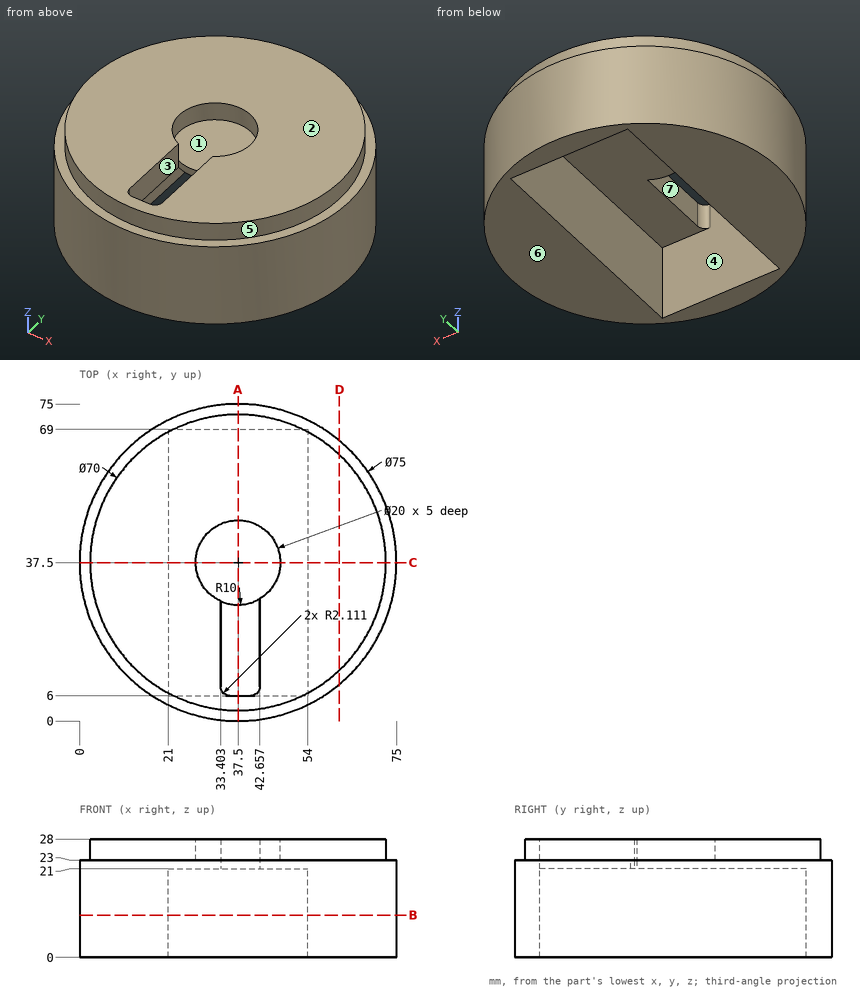
The drawing under review shows one solid part. Ordinate dimensions are in mm from its lowest x, y, z. A direction names the side the tool comes from. Coordinates: 2 decimals unless noted, no trailing zeros. Loops run counter-clockwise (first coordinate to the right, second up) from the corner with the lowest first, then second, coordinate; pieces in that order, holes last. Notation, with made-up numbers: M -40,20 L -14,20 A19 ccw -14,43 Z; hole C 87.25,69.25 d9. An arc over 180 degrees is marked long. Use one line per item in the form item = value.
(1) Consider section A-A (x = 37.5). Write out the cut boundary in (y, z).
Return value:
outline = M 0,0 L 6,0 L 6,28 L 2.5,28 L 2.5,23 L 0,23 Z; M 27.5,21 L 69,21 L 69,0 L 75,0 L 75,23 L 72.5,23 L 72.5,28 L 47.5,28 L 47.5,23 L 27.5,23 Z
(2) Consider section B-B (z = 10). Write out the cut boundary in (x, y), and give its area (3 significant figures).
Return value:
outline = C 37.5,37.5 d75; hole M 21,6 L 54,6 L 54,69 L 21,69 Z
area = 2,340 mm2
(3) Clearance check with flat-ended pins moving along their axes: P1, Ø12, axis at x = 37.5, y = 37.5, coming from the -Z side; P2, Ø2, axis at y = 19, z = 23.5, coming from the +X side (1 decimal); P3, Ø4, axis at y = 52.5, z = 8, coming from the -X side (1 decimal). State where each tip first meets the part, or that it passes through.
Return value:
P1 = 21
P2 = 70.6
P3 = 2.3
(4) Draft analysis for pull direction Y (two halves, no side actions). For the marked faces 5, 6 and 7, state which applies: pulls with the +Y half, pulls with the -Y half, needs draft (parallel to the pull), parting line crosses it, or undercut.
Return value:
face_5 = parting line crosses it
face_6 = needs draft
face_7 = undercut
(5) Consider section C-C (y = 37.5). Write out the cut boundary in (x, z).
Return value:
outline = M 0,0 L 21,0 L 21,21 L 54,21 L 54,0 L 75,0 L 75,23 L 72.5,23 L 72.5,28 L 47.5,28 L 47.5,23 L 27.5,23 L 27.5,28 L 2.5,28 L 2.5,23 L 0,23 Z
(6) Consider section D-D (x = 61.5). Write out the cut boundary in (y, z) (1 decimal).
Return value:
outline = M 8.7,0 L 66.3,0 L 66.3,23 L 63,23 L 63,28 L 12,28 L 12,23 L 8.7,23 Z
(7) For the marked faces 1, 2, 3 and 4, list the 3-axis set-ups (+Z, -Z, +X, -X, +Y, -Y) from which the entire face can be reached by the end or side of a thin tool; tool diameter is ignored.
Return value:
face_1 = +Z
face_2 = +Z, +X, -X, +Y, -Y
face_3 = +Z, -Z
face_4 = -Z
(8) For line 1 along Y through (x, z) = (37.5, 25.45); line 2 along X through (y, z) = (37, 18.5); line 3 along Z through (x, y) = (45.5, 17.5), list the stretches that pass through material, from the lowest coordinate up. Write a range as from..to.
Return value:
line_1 = 2.5..6, 47.5..72.5
line_2 = 0..21, 54..75
line_3 = 21..28
